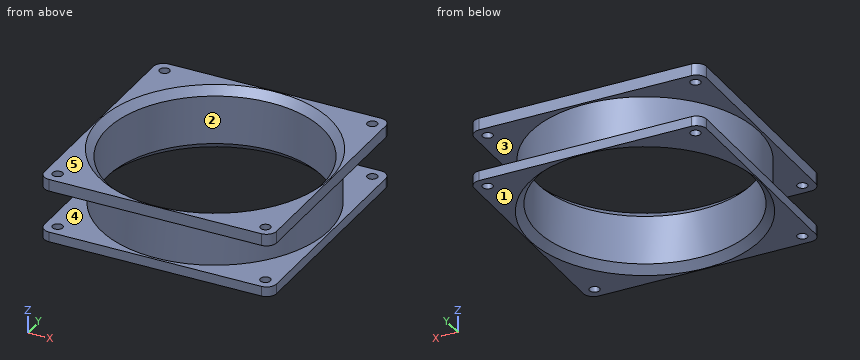
```python
from build123d import *

# Parameters (mm, degrees)
SKETCH_R        = 45
SKETCH_R_2      = 42.5
PAD_DEPTH       = 12.6
SKETCH001_R     = 2
SKETCH001_R_2   = 44.5
PAD001_DEPTH    = 4.7
SKETCH002_R     = 2
SKETCH002_R_2   = 44.5
PAD002_DEPTH    = 3.9
CHAMFER_SIZE    = 3
CHAMFER001_SIZE = 3


with BuildPart() as part:
    # Sketch → Pad (new body, symmetric)
    with BuildSketch(Plane.XY):
        Circle(SKETCH_R)
        Circle(SKETCH_R_2, mode=Mode.SUBTRACT)
    extrude(amount=PAD_DEPTH, both=True)

    # Sketch001 (on Face4 of Pad) → Pad001 (join)
    with BuildSketch(Plane.XY.offset(12.6)):
        with BuildLine():
            Line((-41.85, 45.85), (41.85, 45.85))
            ThreePointArc((45.85, 41.85), (44.678427, 44.678427), (41.85, 45.85))
            Line((45.85, 41.85), (45.85, -41.85))
            ThreePointArc((41.85, -45.85), (44.678427, -44.678427), (45.85, -41.85))
            Line((41.85, -45.85), (-41.85, -45.85))
            ThreePointArc((-45.85, -41.85), (-44.678427, -44.678427), (-41.85, -45.85))
            Line((-45.85, -41.85), (-45.85, 41.85))
            ThreePointArc((-41.85, 45.85), (-44.678427, 44.678427), (-45.85, 41.85))
        make_face()
        with Locations((-41, 41)):
            Circle(SKETCH001_R, mode=Mode.SUBTRACT)
        with Locations((41, 41)):
            Circle(SKETCH001_R, mode=Mode.SUBTRACT)
        with Locations((-41, -41)):
            Circle(SKETCH001_R, mode=Mode.SUBTRACT)
        with Locations((41, -41)):
            Circle(SKETCH001_R, mode=Mode.SUBTRACT)
        Circle(SKETCH001_R_2, mode=Mode.SUBTRACT)
    extrude(amount=-PAD001_DEPTH)

    # Sketch002 (on Face2 of Pad001) → Pad002 (join)
    with BuildSketch(Plane(origin=(0, 0, -12.6), x_dir=(1, 0, 0), z_dir=(0, 0, -1))):
        with BuildLine():
            Line((-41.85, 45.85), (41.85, 45.85))
            ThreePointArc((45.85, 41.85), (44.678427, 44.678427), (41.85, 45.85))
            Line((45.85, 41.85), (45.85, -41.85))
            ThreePointArc((41.85, -45.85), (44.678427, -44.678427), (45.85, -41.85))
            Line((41.85, -45.85), (-41.85, -45.85))
            ThreePointArc((-45.85, -41.85), (-44.678427, -44.678427), (-41.85, -45.85))
            Line((-45.85, -41.85), (-45.85, 41.85))
            ThreePointArc((-41.85, 45.85), (-44.678427, 44.678427), (-45.85, 41.85))
        make_face()
        with Locations((-41, 41)):
            Circle(SKETCH002_R, mode=Mode.SUBTRACT)
        with Locations((41, 41)):
            Circle(SKETCH002_R, mode=Mode.SUBTRACT)
        with Locations((-41, -41)):
            Circle(SKETCH002_R, mode=Mode.SUBTRACT)
        with Locations((41, -41)):
            Circle(SKETCH002_R, mode=Mode.SUBTRACT)
        Circle(SKETCH002_R_2, mode=Mode.SUBTRACT)
    extrude(amount=-PAD002_DEPTH)

    # Chamfer
    chamfer_edges = [part.edges().sort_by_distance(p)[0] for p in [
        (-42.5, 0, 12.6),
    ]]
    chamfer(chamfer_edges, length=CHAMFER_SIZE)

    # Chamfer001
    chamfer001_edges = [part.edges().sort_by_distance(p)[0] for p in [
        (-42.5, 0, -12.6),
    ]]
    chamfer(chamfer001_edges, length=CHAMFER001_SIZE)


solid = part.part
```
Input: part model. Units: mm. Frame: model coordinates. Face numbers are marked on the shaded views. A direction names the side the tool comes from. Give positions to 0.01 mm unless a question says otherwise; leave off trailing zeros. Order: outer loops, then holes, each group sorted by start corner. A loop starts at its lowest first (then second) coordinate and runs counter-clockwise, first axis right, second up.
1. Line query: probe 1 along Z at (x, y) = (26.5, 38); probe 2 along Y at (x, z) = (-0.5, 9.25); probe 3 along X at (y, z) = (7.5, 9.25). Output: solid intervals per line, ascending.
Computed:
probe 1: z = -12.6 to -8.7, 7.9 to 12.6
probe 2: y = -45.85 to -42.5, 42.5 to 45.85
probe 3: x = -45.85 to -41.83, 41.83 to 45.85
2. Set-up query: the marked faces 4 and 5. Return all of +Z, -Z, +X, -X, +Y, -Y with unobstructed straight access to the full face (end or side cutting, diameter ignored); none if empty.
Computed:
face 4: none
face 5: +Z, +X, -X, +Y, -Y
3. Cut plane D-D (z = -4.75). Return loops of the section in (x, y), and give its area (3 significant figures).
Computed:
outline: circle Ø90 at (0, 0); hole circle Ø85 at (0, 0)
area: 687 mm2
4. Draft query along Z for the marked faces 1, 2 and 3. Return one class per face: released by +Z, released by -Z, zero draft, split by the parting line, or undercut.
Computed:
face 1: released by -Z
face 2: zero draft
face 3: undercut
5. Cut plane B-B (z = 10.75). Return loops of the section in (x, y).
Computed:
outline: (-45.85, -41.85) arc R4 ccw to (-41.85, -45.85) - (41.85, -45.85) arc R4 ccw to (45.85, -41.85) - (45.85, 41.85) arc R4 ccw to (41.85, 45.85) - (-41.85, 45.85) arc R4 ccw to (-45.85, 41.85) - close; hole circle Ø87.3 at (0, 0); hole circle Ø4 at (-41, -41); hole circle Ø4 at (-41, 41); hole circle Ø4 at (41, -41); hole circle Ø4 at (41, 41)
6. Cut plane A-A (y = 0). Return loops of the section in (x, z).
Computed:
outline: (-45.85, -12.6) - (-45.5, -12.6) - (-42.5, -9.6) - (-42.5, 9.6) - (-45.5, 12.6) - (-45.85, 12.6) - (-45.85, 7.9) - (-45, 7.9) - (-45, -8.7) - (-45.85, -8.7) - close; (42.5, -9.6) - (45.5, -12.6) - (45.85, -12.6) - (45.85, -8.7) - (45, -8.7) - (45, 7.9) - (45.85, 7.9) - (45.85, 12.6) - (45.5, 12.6) - (42.5, 9.6) - close
7. Pin query (flat end, axial travel): pin 1 Ø3 at (y, z) = (13.5, -4.5) entering from +X; pin 2 Ø4 at (y, z) = (26, 3.5) entering from +X; pin 3 Ø1 at (x, z) = (-5.5, -2) entering from -Y. Return the tip coordinate at first contact, or that it passes through.
Computed:
pin 1: stops at x = 43.37
pin 2: stops at x = 38.07
pin 3: stops at y = -44.72
